Work out the finished part from the listing and answer in its coordinate system (mm). Face numbers are marked on the shaded views. A direction names the side the tool comes from. Coordinates: 2 decimals unless noted, no trailing zeros. Order: outer loops, then holes, each group sorted by start corner. A loop starts at its lowest first (then second) coordinate and runs counter-clockwise, first axis right, second up. Notation, with made-up numbers: M 89.5,32.5 L 127.5,32.5 A18 ccw 127.5,67.5 Z; hole C 37.5,-16.75 d10. An arc over 180 degrees is marked long. Use a Markdown table: item, result.
Autodesk Inventor part; units mm, degrees
ref_plane "YZ Plane" through (0, 0, 0) normal (1, 0, 0) x (0, 1, 0)
ref_plane "XZ Plane" through (0, 0, 0) normal (0, 1, 0) x (-1, 0, 0)
ref_plane "XY Plane" through (0, 0, 0) normal (0, 0, 1) x (1, 0, 0)
sketch "Sketch1" plane through (0, 0, 0) normal (1, 0, 0) x (0, 1, 0)
  line L0 (0, 17.78) -> (3.175, 17.78)
  line L1 (3.175, 17.78) -> (3.175, 13.462)
  line L2 (0, 0) -> (30.099, 0)
  line L3 (30.099, 0) -> (30.099, 3.2908)
  line L4 (30.099, 3.2908) -> (23.7557, 3.2908)
  line L5 (23.7557, 3.2908) -> (3.175, 13.462)
  line L6 (23.7557, 0) -> (0, 13.462)
  line L7 (0, 17.78) -> (0, 13.462)
  dimension "d0" = 17.78
  dimension "d1" = 3.175
  dimension "d2" = 4.318
  dimension "d3" = 30.099
revolve "Revolution1" add sketch "Sketch1" angle 360 about axis through (0, 0, 0) along (0, 1, 0)
properties part number "nozzletopcone"
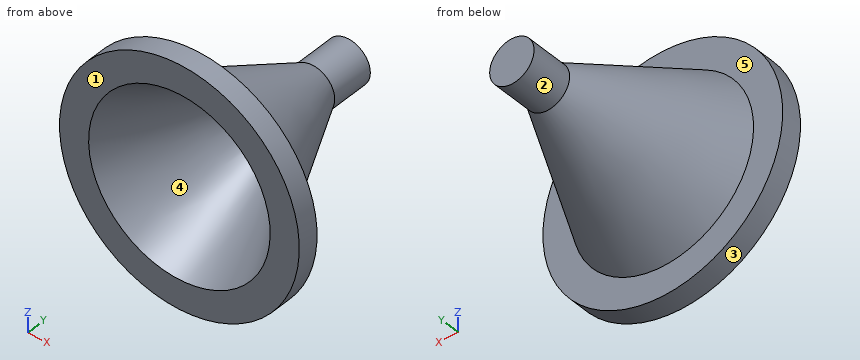
(1) Which of the six approach directions +Z, -Z, +X, -X, +Y, -Y give full straight-line access (tool end or side, diameter ignored) to the marked faces 1 and 2?
Conclusion:
| item | result |
|---|---|
| face 1 | +Z, -Z, +X, -X, -Y |
| face 2 | +Y |
(2) A cutting plane is placed at B-B (y = 8). Determine the outline of the cut face in (x, z).
Conclusion:
| item | result |
|---|---|
| outline | C 0,0 d22.15; hole C 0,0 d17.86 |
(3) Given P1, Ø10, axis at x = 3.5, y = 25, coming from the +Z side; P2, Ø1.5, axis at x = -6.5, z = 6.5, coming from the -Y side; P3, Ø4, axis at x = 9, z = 0, coming from the -Y side, each flat-ended and moving along its own axis, determine where each tip first touches the part or whether it passes through.
Conclusion:
| item | result |
|---|---|
| P1 | z = 4.72 |
| P2 | y = 6.21 |
| P3 | y = 4.34 |
(4) Determine the mould class of the marked faces 3, 4 and 5 for opening direction Z: pulls with the +Z half, pulls with the -Z half, needs draft (parallel to the pull), parting line crosses it, or undercut.
Conclusion:
| item | result |
|---|---|
| face 3 | parting line crosses it |
| face 4 | undercut |
| face 5 | needs draft |
(5) A cutting plane is placed at D-D (y = 18). Determine the outline of the cut face in (x, z), then the cut area to 3 significant figures.
Conclusion:
| item | result |
|---|---|
| outline | C 0,0 d12.27; hole C 0,0 d6.52 |
| area | 84.8 mm2 |
(6) A cutting plane is placed at C-C (z = -14.5). Determine the outline of the cut face in (x, y) (3 decimals).
Conclusion:
| item | result |
|---|---|
| outline | M -10.29,0 L 10.29,0 L 10.29,3.175 L -10.29,3.175 Z |
(7) A cutting plane is placed at A-A (y = 27.5). Determine the outline of the cut face in (x, z), then the cut area to 3 significant figures.
Conclusion:
| item | result |
|---|---|
| outline | C 0,0 d6.58 |
| area | 34.0 mm2 |
(8) Straight lines are drawn through the part: L1, parallel to Y at x = -15, z = 8 (3 decimals); L2, parallel to Z at x = -4, y = 8; L3, parallel to X at y = 4, z = 2.5. For each, find the intervals that lie inside material, in ascending order.
Conclusion:
| item | result |
|---|---|
| L1 | 0 to 3.175 |
| L2 | -10.33 to -7.98, 7.98 to 10.33 |
| L3 | -12.81 to -10.91, 10.91 to 12.81 |
